from build123d import *

# Parameters (mm, degrees)
F0_R     = 7.5
F1_DEPTH = 4
F2_R     = 5
F3_DEPTH = 100
F4_W     = 4
F4_H     = 4
F5_DEPTH = 20
F6_R     = 1.5
F7_DEPTH = 122.4


with BuildPart() as f1:
    # F0 (on Top) → F1 (new body)
    with BuildSketch(Plane.XY):
        Circle(F0_R)
    extrude(amount=F1_DEPTH)

    # F2 (on Top) → F3 (join)
    with BuildSketch(Plane.XY):
        Circle(F2_R)
    extrude(amount=F3_DEPTH)

    # F4 (on face) → F5 (join)
    with BuildSketch(Plane.XY.offset(100)):
        Rectangle(F4_W, F4_H)
    extrude(amount=F5_DEPTH)

    # F6 (on face) → F7 (cut)
    with BuildSketch(Plane(origin=(0, 0, 0), x_dir=(1, 0, 0), z_dir=(0, 0, -1))):
        Circle(F6_R)
    extrude(amount=-F7_DEPTH, mode=Mode.SUBTRACT)


solid = f1.part
Can you work these out from the model? Positions are in its coordinate system, mm. A direction names the side the tool comes from. Give positions to 0.01 mm unless a question says otherwise; leave off trailing zeros. Loops run counter-clockwise (first coordinate to the right, second up) from the corner with the lowest first, then second, coordinate; pieces in that order, holes last. Notation, with made-up numbers: M 4,-3 L 55,-3 A12 ccw 55,5 Z; hole C 89.25,-9 d4. An arc over 180 degrees is marked long. One line per item, written item: value.
1) On a 3-axis mill with a long thin cutter (end or side, diameter ignored), from which of +Z, -Z, +X, -X, +Y, -Y can I reach the whole of each face in a straight line? I mean faces 1 (the face through (0, 2, 110)), 2 (the face through (2, -5, 4)), 3 (the face through (-2, 0, 110)), 4 (the face through (2, 0, 110)), 5 (the face through (0, -2, 110)). Say none if no direction works.
Geometry check:
face 1: +Z, +X, -X, +Y
face 2: +Z
face 3: +Z, -X, +Y, -Y
face 4: +Z, +X, +Y, -Y
face 5: +Z, +X, -X, -Y
2) Imagine slicing it at C-C on z = 112. Write out the boundary of the cut face in (x, y).
Geometry check:
outline: M -2,-2 L 2,-2 L 2,2 L -2,2 Z; hole C 0,0 d3
3) Thinking about a two-plate mould opening in Y: for faces 6 (the face through (0.9, 1.4, 120)), 7 (the face through (-1.5, -0.07, 59.16)), 8 (the face through (-1.08, -4.88, 51.33)), which applies, +Y half, -Y half, draft (parallel to the pull), parting line (faces both ways), or undercut?
Geometry check:
face 6: draft
face 7: undercut
face 8: parting line
4) Imagine slicing it at D-D on z = 47. Write out the boundary of the cut face in (x, y).
Geometry check:
outline: C 0,0 d10; hole C 0,0 d3
5) Please list where these lines run through material, in increasing order: line 1 (X direction, y = 0, z = 46); line 2 (Z direction, x = -0.25, y = -3.75).
Geometry check:
line 1: x = -5 to -1.5, 1.5 to 5
line 2: z = 0 to 100
6) Imagine slicing it at A-A on y = 0. Write out the boundary of the cut face in (x, z).
Geometry check:
outline: M -7.5,0 L -1.5,0 L -1.5,120 L -2,120 L -2,100 L -5,100 L -5,4 L -7.5,4 Z; M 1.5,0 L 7.5,0 L 7.5,4 L 5,4 L 5,100 L 2,100 L 2,120 L 1.5,120 Z
7) I'm going to push flat-ended pins straight in: pin 1 (1.5 mm diameter, centred on x = 2.5, z = 69, fed in from -Y); pin 2 (1.2 mm diameter, centred on x = 0.5, z = 110, fed in from -Y); pin 3 (4 mm diameter, centred on x = -3, z = 80, fed in from +Y). Where does each tip first touch, or does it pass through?
Geometry check:
pin 1: stops at y = -4.68
pin 2: stops at y = -2
pin 3: stops at y = 4.9
